Here's how the part is built. I have some questions about the finished solid (model axes, mm). A direction names the side the tool comes from. Round coordinates to 2 decimals unless told otherwise and drop trailing zeros. Write each loop counter-clockwise with the first axis right and the second up, starting at its lowest first coordinate (ties: lowest second). Pieces come first, ordered by that corner, then holes. Notation, with made-up numbers: (-38, -0.5) -> (-32, -0.5) arc R26 cw to (-32, 35.5) -> close; hole circle Ø4 at (14, -24.5). An arc over 180 degrees is marked (long way). Put each result on its own line as item: value. Start each with the question number.
1) If I drill on line 1 along X through (y, z) = (3, 0.3); line 2 along Y through (x, z) = (-42, 1.6); line 3 along X through (y, z) = (11, 0.1), over which ranges is the centre line in solid material (lowest first)? Write a range as [from, to].
2) Which directions (+Z, -Z, +X, -X, +Y, -Y) give clear straight access to the entire face, cutting with the end or side of a thin tool? Please do faces 4 (the flat face through (-13.532, -23.547, 1.507)), 5 (the flat face through (-23.47, -10.03, 1.49)), 6 (the flat face through (79, 0, 2)).
3) We'd pull the mould along Y, two halves only. Please class faces 1 (the flat face through (32.008, -16.225, 0.493)), 2 (the flat face through (0, 0, 2)), 3 (the flat face through (33.541, 3.668, 1.507)): released by +Y, released by -Y, zero draft, split by the parting line, or undercut.
4) Will these pins go through, and if not, where does the flat tip stop? P1, Ø0.6, axis at y = 0.5, z = 1.5, coming from the +X side; P2, Ø1.1, axis at x = -66, z = 0.5, coming from the +Y side; P3, Ø6, axis at x = -78.5, y = -21, coming from the +Z side; P4, Ø12, axis at x = -0.5, y = 0.5, coming from the -Z side.
5) I want a section at A-A, the plane z = 0.45. List the corners of the cut face in (x, y) for me, then the cut area to 3 significant figures.
from build123d import *

# Parameters (mm, degrees)
F1_DEPTH  = 2
F3_DEPTH  = 2
F5_DEPTH  = 2
F7_DEPTH  = 2
F9_DEPTH  = 1
F10_SIZE  = 0.99999
F11_W     = 3
F11_H     = 10
F12_DEPTH = 2


# Not quite as in the source:
# - a fillet or chamfer is up to 0.001 mm smaller than in the source, because OpenCascade refuses the exact size


with BuildPart() as f1:
    # F0 (on Top) → F1 (new body)
    with BuildSketch(Plane.XY):
        Polygon((37.9150851114, 8), (28.3810563706, 0), (37.9150851114, -8), (130, -8), (130, 0), (130, 8), align=None)
    extrude(amount=F1_DEPTH)



with BuildPart() as f1b:
    # F0 (on Top) → F1, piece 2 (new body)
    with BuildSketch(Plane.XY):
        Polygon((-37.9150851114, -8), (-28.3810563706, 0), (-37.9150851114, 8), (-130, 8), (-130, 0), (-130, -8), align=None)
    extrude(amount=F1_DEPTH)


with BuildPart() as f3:
    # F2 (on Top) → F3 (new body)
    with BuildSketch(Plane.XY):
        Polygon((-37.8240925528, 8.25), (0, -23.4881821107), (37.8240925528, 8.25), (130, 8.25), (130, 18.25), (34.1843902102, 18.25), (0, -10.4341092174), (-34.1843902102, 18.25), (-130, 18.25), (-130, 8.25), align=None)
    extrude(amount=F3_DEPTH)


with BuildPart() as f5:
    # F4 (on Top) → F5 (new body)
    with BuildSketch(Plane.XY):
        Polygon((12.4810478052, 0.365085215), (21.6735811226, 8.0785365312), (0, 26.2648304575), (-21.6735811226, 8.0785365312), (-12.4810478052, 0.365085215), (0, 10.8379278251), align=None)
    extrude(amount=F5_DEPTH)


with BuildPart() as f5b:
    # F4 (on Top) → F5, piece 2 (new body)
    with BuildSketch(Plane.XY):
        Polygon((37.8240925528, -8.25), (28.1865908923, -0.1631759112), (20.5261464611, -6.591052008), (34.4207396164, -18.25), (130, -18.25), (130, -8.25), align=None)
    extrude(amount=F5_DEPTH)


with BuildPart() as f5c:
    # F4 (on Top) → F5, piece 3 (new body)
    with BuildSketch(Plane.XY):
        Polygon((-130, -18.25), (-34.4207396164, -18.25), (-20.5261464611, -6.591052008), (-28.1865908923, -0.1631759112), (-37.8240925528, -8.25), (-130, -8.25), align=None)
    extrude(amount=F5_DEPTH)


with BuildPart() as f7:
    # F6 (on Top) → F7 (new body)
    with BuildSketch(Plane.XY):
        Polygon((-27.3324382036, -12.6285607212), (0, -35.563199537), (27.3324382036, -12.6285607212), (20.3316809827, -6.7542279192), (0, -23.814533933), (-20.3316809827, -6.7542279192), align=None)
    extrude(amount=F7_DEPTH)


with BuildPart() as f7b:
    # F6 (on Top) → F7, piece 2 (new body)
    with BuildSketch(Plane.XY):
        Polygon((-12.2865823268, 0.2019093038), (0, -10.107757395), (12.2865823268, 0.2019093038), (0, 10.5115760027), align=None)
    extrude(amount=F7_DEPTH)


with BuildPart() as f1_1:
    add(f1.part)

    add(f1b.part)  # F9 merges F1b

    add(f3.part)  # F9 merges F3

    add(f5.part)  # F9 merges F5

    add(f5b.part)  # F9 merges F5b

    add(f5c.part)  # F9 merges F5c

    add(f7.part)  # F9 merges F7

    add(f7b.part)  # F9 merges F7b
    # F8 (on Top) → F9 (join)
    with BuildSketch(Plane.XY):
        Polygon((21.868046601, 7.9153606201), (0, 26.2648304575), (-21.868046601, 7.9153606201), (-34.1843902102, 18.25), (-130, 18.25), (-130, -18.25), (-34.4207396164, -18.25), (-27.526903682, -12.46538481), (0, -35.563199537), (27.526903682, -12.46538481), (34.4207396164, -18.25), (130, -18.25), (130, 18.25), (34.1843902102, 18.25), align=None)
    extrude(amount=F9_DEPTH)

    # F10 (size 1 in the source; OpenCascade refuses exactly that, so slightly less here)
    f10_edges = [f1_1.edges().sort_by_distance(p)[0] for p in [
        (-18.912046, -7.619091, 2),
        (18.912046, -7.619091, 2),
        (83.912046, 8.25, 2),
        (130, 13.25, 2),
        (82.092195, 18.25, 2),
        (17.092195, 3.907945, 2),
        (-17.092195, 3.907945, 2),
        (-82.092195, 18.25, 2),
        (-130, 13.25, 2),
        (-83.912046, 8.25, 2),
        (-33.148071, -4, 2),
        (-33.148071, 4, 2),
        (-83.957543, 8, 2),
        (-130, 0, 2),
        (-83.957543, -8, 2),
        (-83.912046, -8.25, 2),
        (-130, -13.25, 2),
        (-82.21037, -18.25, 2),
        (-27.473443, -12.420526, 2),
        (-24.356369, -3.377114, 2),
        (-33.005342, -4.206588, 2),
        (6.240524, 5.601507, 2),
        (17.077314, 4.221811, 2),
        (10.836791, 17.171683, 2),
        (-10.836791, 17.171683, 2),
        (-17.077314, 4.221811, 2),
        (-6.240524, 5.601507, 2),
        (-6.143291, -4.952924, 2),
        (6.143291, -4.952924, 2),
        (6.143291, 5.356743, 2),
        (-6.143291, 5.356743, 2),
        (-23.83206, -9.691394, 2),
        (-13.666219, -24.09588, 2),
        (13.666219, -24.09588, 2),
        (23.83206, -9.691394, 2),
        (10.16584, -15.284381, 2),
        (-10.16584, -15.284381, 2),
        (33.005342, -4.206588, 2),
        (24.356369, -3.377114, 2),
        (27.473443, -12.420526, 2),
        (82.21037, -18.25, 2),
        (130, -13.25, 2),
        (83.912046, -8.25, 2),
        (33.148071, 4, 2),
        (33.148071, -4, 2),
        (83.957543, -8, 2),
        (130, 0, 2),
        (83.957543, 8, 2),
    ]]
    chamfer(f10_edges, length=F10_SIZE)

    # F11 (on face) → F12 (cut, through all)
    with BuildSketch(Plane.XY.offset(2)):
        with Locations((123.5, 0)):
            Rectangle(F11_W, F11_H)
        with Locations((-123.5, 0)):
            Rectangle(F11_W, F11_H)
    extrude(amount=-F12_DEPTH, mode=Mode.SUBTRACT)


solid = f1_1.part
Findings:
1. line 1: x = [-130, -125], [-122, 122], [125, 130]
1. line 2: y = [-17.65, -8.85], [-7.4, 7.4], [8.85, 17.65]
1. line 3: x = [-130, -25.54], [-18.19, 18.19], [25.54, 130]
2. face 4: +Z, -Y
2. face 5: +Z
2. face 6: +Z, +X, -X, +Y, -Y
3. face 1: released by -Y
3. face 2: zero draft
3. face 3: undercut
4. P1: stops at x = 129.8
4. P2: stops at y = 18.25
4. P3: stops at z = 1.25
4. P4: stops at z = 0
5. outline: (-130, -18.25) -> (-34.42, -18.25) -> (-27.53, -12.47) -> (0, -35.56) -> (27.53, -12.47) -> (34.42, -18.25) -> (130, -18.25) -> (130, 18.25) -> (34.18, 18.25) -> (21.87, 7.92) -> (0, 26.26) -> (-21.87, 7.92) -> (-34.18, 18.25) -> (-130, 18.25) -> close; hole (-125, -5) -> (-122, -5) -> (-122, 5) -> (-125, 5) -> close; hole (122, -5) -> (125, -5) -> (125, 5) -> (122, 5) -> close
5. area: 9,530 mm2
